Part model, mm, in its own coordinate system. Give positions to 0.01 mm unless a question says otherwise; leave off trailing zeros. Order: outer loops, then holes, each group sorted by start corner. A loop starts at its lowest first (then second) coordinate and runs counter-clockwise, first axis right, second up. Notation, with made-up numbers: (68.25, 62) - (102.25, 62) arc R18 cw to (102.25, 90) - close; hole circle Ø5 at (23, 25.5). An arc over 180 degrees is marked (long way). One line per item, written item: value.
```python
from build123d import *

# Parameters (mm, degrees)
SKETCH1_W            = 227.084
SKETCH1_H            = 106.85
BOSS_EXTRUDE1_DEPTH  = 10
SKETCH2_R            = 10.65
CUT_EXTRUDE1_DEPTH   = 22.3
LPATTERN1_COUNT      = 4
LPATTERN1_PITCH      = 23.3
LPATTERN1_COUNT_DIR2 = 6
LPATTERN1_PITCH_DIR2 = 40.356783816
SKETCH6_R            = 10.65
CUT_EXTRUDE2_DEPTH   = 252.165414729
LPATTERN2_COUNT      = 4
LPATTERN2_PITCH      = 23.3
LPATTERN2_COUNT_DIR2 = 5
LPATTERN2_PITCH_DIR2 = 40.356783816


with BuildPart() as part:
    # Sketch1 → Boss-Extrude1 (new body)
    with BuildSketch(Plane(origin=(0, 0, 0), x_dir=(1, 0, 0), z_dir=(0, 1, 0))):
        with Locations((113.542, 53.425)):
            Rectangle(SKETCH1_W, SKETCH1_H)
    extrude(amount=BOSS_EXTRUDE1_DEPTH)

    # Sketch2 → Cut-Extrude1 (cut)
    with BuildSketch(Plane(origin=(0, 10, 0), x_dir=(1, 0, 0), z_dir=(0, 1, 0))):
        with Locations(Location((12.65, 12.65, 0), (0, 0, 270))):
            Circle(SKETCH2_R)
    cut_extrude1 = extrude(amount=-CUT_EXTRUDE1_DEPTH, mode=Mode.SUBTRACT)

    # LPattern1: Cut-Extrude1 4 × 6
    with Locations(*[(j * LPATTERN1_PITCH_DIR2, 0, -i * LPATTERN1_PITCH) for i in range(LPATTERN1_COUNT) for j in range(LPATTERN1_COUNT_DIR2) if (i, j) != (0, 0)]):
        add(cut_extrude1, mode=Mode.SUBTRACT)

    # Sketch6 → Cut-Extrude2 (cut, through all)
    with BuildSketch(Plane(origin=(0, 10, 0), x_dir=(1, 0, 0), z_dir=(0, 1, 0))):
        with Locations(Location((32.828391908, 24.3, 0), (0, 0, 270))):
            Circle(SKETCH6_R)
    cut_extrude2 = extrude(amount=-CUT_EXTRUDE2_DEPTH, mode=Mode.SUBTRACT)

    # LPattern2: Cut-Extrude2 4 × 5
    with Locations(*[(j * LPATTERN2_PITCH_DIR2, 0, -i * LPATTERN2_PITCH) for i in range(LPATTERN2_COUNT) for j in range(LPATTERN2_COUNT_DIR2) if (i, j) != (0, 0)]):
        add(cut_extrude2, mode=Mode.SUBTRACT)


solid = part.part
```
1) Cut at B-B, the plane z = -29.5. Give the number of separate pieces and of enclosed holes in the cut face, then the cut area to 3 significant figures.
Outcome:
separate pieces: 12
enclosed holes: 0
area: 324 mm^2
2) Cut at A-A, the plane x = 12.65. Give the cut face in (y, z).
Outcome:
outline: (0, -106.85) - (10, -106.85) - (10, -93.2) - (0, -93.2) - close; (0, -71.9) - (10, -71.9) - (10, -69.9) - (0, -69.9) - close; (0, -48.6) - (10, -48.6) - (10, -46.6) - (0, -46.6) - close; (0, -25.3) - (10, -25.3) - (10, -23.3) - (0, -23.3) - close; (0, -2) - (10, -2) - (10, 0) - (0, 0) - close
3) Cut at D-D, the plane x = 199. Give the cut face in (y, z).
Outcome:
outline: (0, -106.85) - (10, -106.85) - (10, -103.73) - (0, -103.73) - close; (0, -84.67) - (10, -84.67) - (10, -80.43) - (0, -80.43) - close; (0, -61.37) - (10, -61.37) - (10, -57.13) - (0, -57.13) - close; (0, -38.07) - (10, -38.07) - (10, -33.83) - (0, -33.83) - close; (0, -14.77) - (10, -14.77) - (10, 0) - (0, 0) - close
4) Drill centre lines: line 1 along Z through (x, y) = (53.5, 2.75); line 2 along Z through (x, y) = (114, 9.5); line 3 along X through (y, z) = (5, -94.2). Where is each one in solid material? Low to high. Write a range as from..to.
Outcome:
line 1: z = -106.85..-93.19, -71.91..-69.89, -48.61..-46.59, -25.31..-23.29, -2.01..0
line 2: z = -106.85..-104.84, -83.56..-81.54, -60.26..-58.24, -36.96..-34.94, -13.66..0
line 3: x = 0..22.18, 43.48..62.54, 83.84..102.89, 124.19..143.25, 164.55..183.61, 204.91..227.08
5) Mould opens along X. For faces 1 (the flat face through (112, 5, -106.85)), 2 (the cylindrical face through (86.88, 5.07, -91)), 3 (the flat face through (0, 5, -53)) say: released by +X, released by -X, zero draft, split by the parting line, or undercut.
Outcome:
face 1: zero draft
face 2: undercut
face 3: released by -X
6) Pin check, flat tip, straight feed: pin 1 (3 mm diameter, centred on x = 95, z = -21, fed in from -Y). Stop position of the tip, or through.
Outcome:
pin 1: passes through
